Read the model definition and answer for the solid it produces. Units are mm, in the model's axes. Face numbers are marked on the shaded views. A direction names the side the tool comes from. Give positions to 0.01 mm unless a question says otherwise; leave off trailing zeros. Order: outer loops, then holes, each group sorted by start corner. A loop starts at its lowest first (then second) coordinate and runs counter-clockwise, first axis right, second up. Notation, with made-up numbers: M 40,86.25 L 55,86.25 A33 cw 55,122.25 Z; hole C 10,25 d4. An arc over 180 degrees is marked long. Write item = value, one per line. Start each with the question number.
from build123d import *

# Parameters (mm, degrees)
F0_W     = 25.4
F0_H     = 25.4
F1_DEPTH = 25.4
F2_W     = 20.32
F2_H     = 22.86
F3_DEPTH = 7.62
F4_W     = 3.556
F4_H     = 20.32
F5_DEPTH = 3.048
F6_W     = 3.556
F6_H     = 19.812
F7_DEPTH = 3.048
F8_W     = 3.556
F8_H     = 19.812
F9_DEPTH = 3.048


with BuildPart() as f1:
    # F0 (on Top) → F1 (new body)
    with BuildSketch(Plane.XY):
        Rectangle(F0_W, F0_H)
    extrude(amount=F1_DEPTH)

    # F2 (on face) → F3 (join)
    with BuildSketch(Plane(origin=(-12.7, 0, 0), x_dir=(0, -1, 0), z_dir=(-1, 0, 0))):
        with Locations((0, 11.43)):
            Rectangle(F2_W, F2_H)
    extrude(amount=F3_DEPTH)

    # F4 (on face) → F5 (cut)
    with BuildSketch(Plane.XY.offset(22.86)):
        with Locations((-16.51, 0)):
            Rectangle(F4_W, F4_H)
    extrude(amount=-F5_DEPTH, mode=Mode.SUBTRACT)

    # F6 (on face) → F7 (cut)
    with BuildSketch(Plane.XZ.offset(10.16)):
        with Locations((-16.51, 9.906)):
            Rectangle(F6_W, F6_H)
    extrude(amount=-F7_DEPTH, mode=Mode.SUBTRACT)

    # F8 (on face) → F9 (cut)
    with BuildSketch(Plane(origin=(0, 10.16, 0), x_dir=(-1, 0, 0), z_dir=(0, 1, 0))):
        with Locations((16.51, 9.906)):
            Rectangle(F8_W, F8_H)
    extrude(amount=-F9_DEPTH, mode=Mode.SUBTRACT)


with BuildPart() as f10_1:
    # F10: copy of F1
    add(f1.part.moved(Location((-54.102, 0, 0))))


solid = f1.part
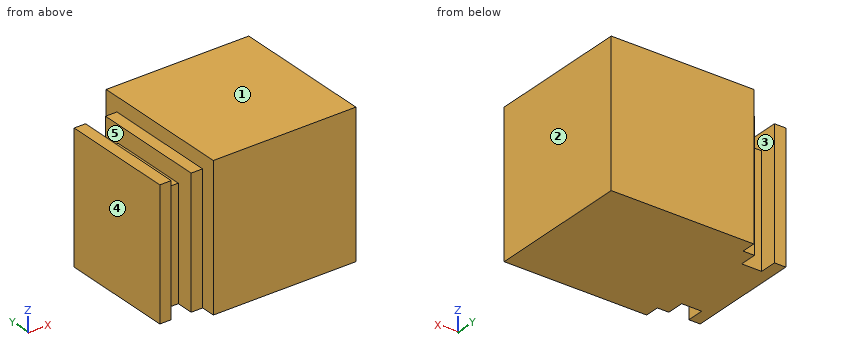
1) For the marked faces 4 and 5, determine the directions among +Z, -Z, +X, -X, +Y, -Y from which every point of the face is accessible in a straight line to the end or side of a thin tool.
2) Find section D-D on z = 23.75. Determine the outline of the cut face in (x, y), plus the area to 3 significant figures.
3) Each of these flat-tipped pins is pushed along its axis until it touches: P1, Ø2, axis at x = -19.5, z = 8, coming from the -Y side; P2, Ø3, axis at x = -17, y = 1.5, coming from the +Z side; P3, Ø1, axis at x = -19.5, z = 17, coming from the +Y side. Where does it stop, or does it pass through?
4) Find section A-A on y = 9.5. Determine the outline of the cut face in (x, z).
5) Find the intervals of material crossed by probe 1 along X at (y, z) = (-8.25, 12.75); probe 2 along Z at (x, y) = (-16, 5.75); probe 3 along Z at (x, y) = (-19, 7), in increasing order. Write a range as [from, to].
6) Find section C-C on z = 3.5. Determine the outline of the cut face in (x, y), plus the area to 3 significant figures.
7) Find section B-B on y = 2. Determine the outline of the cut face in (x, z).
8) For a pull along X with two mould halves and no side action, classify the marked faces 1, 2 and 3 as pulls with the +X half, pulls with the -X half, needs draft (parallel to the pull), parting line crosses it, or undercut.
Numbers:
q1.face_4 = +Z, -Z, -X, +Y, -Y
q1.face_5 = +Z
q2.outline = M -12.7,-12.7 L 12.7,-12.7 L 12.7,12.7 L -12.7,12.7 Z
q2.area = 645 mm2
q3.P1 = -10.16
q3.P2 = 22.86
q3.P3 = 10.16
q4.outline = M -20.32,0 L -18.29,0 L -18.29,22.86 L -20.32,22.86 Z; M -14.73,0 L 12.7,0 L 12.7,25.4 L -12.7,25.4 L -12.7,22.86 L -14.73,22.86 Z
q5.probe_1 = [-20.32, -18.29], [-14.73, 12.7]
q5.probe_2 = [0, 19.81]
q5.probe_3 = [0, 22.86]
q6.outline = M -20.32,-10.16 L -18.29,-10.16 L -18.29,-7.11 L -14.73,-7.11 L -14.73,-10.16 L -12.7,-10.16 L -12.7,-12.7 L 12.7,-12.7 L 12.7,12.7 L -12.7,12.7 L -12.7,10.16 L -14.73,10.16 L -14.73,7.11 L -18.29,7.11 L -18.29,10.16 L -20.32,10.16 Z
q6.area = 778 mm2
q7.outline = M -20.32,0 L 12.7,0 L 12.7,25.4 L -12.7,25.4 L -12.7,22.86 L -14.73,22.86 L -14.73,19.81 L -18.29,19.81 L -18.29,22.86 L -20.32,22.86 Z
q8.face_1 = needs draft
q8.face_2 = pulls with the +X half
q8.face_3 = undercut
